Verification items for this drawing (mm, ordinates from the low corner). A direction names the side the tool comes from. Round coordinates to 2 decimals unless told otherwise and drop trailing zeros. Order: outer loops, then holes, each group sorted by start corner. A loop starts at its lowest first (then second) coordinate and runs counter-clockwise, first axis right, second up. Notation, with made-up numbers: (61, 29.25) - (67, 29.25) arc R14 cw to (67, 50.25) - close; hole circle Ø2 at (14.25, 42.25). An arc over 180 degrees is marked (long way). Use a Markdown table: item, result. Add a question column.
(1) Section check B-B on y = 39.5. Record the boundary of the cut face in (x, z).
(2) Section check D-D on x = 31. Record the boundary of the cut face in (y, z).
(3) Gauge pin test, flat ends, axial feed: P1, Ø1.5, axis at y = 55.5, z = 19, coming from the +X side; P2, Ø3, axis at x = 38, y = 24, coming from the -Z side. Record the tip position at first contact, or that the pin passes through.
(4) Mould release check, pull along Y, two halves, no side actions. Record for the marked faces 3, 4 and 5: released by +Y, released by -Y, zero draft, split by the parting line, or undercut.
(5) Section check C-C on z = 2.75. Record the boundary of the cut face in (x, y).
(6) Thickness scan on line 1 along Z through (x, y) = (31, 1); line 2 along Y through (x, z) = (12, 3.5); line 3 along Y through (x, z) = (5, 22.35). Record the ranges inside material, lowest first. Write a range as [from, to].
(7) Section check A-A on x = 7.5. Record the boundary of the cut face in (y, z).
(8) Access from +Z, -Z, +X, -X, +Y, -Y to the whole of each face (thin tool, end or side, straight path). Record for the marked faces 1 and 2.
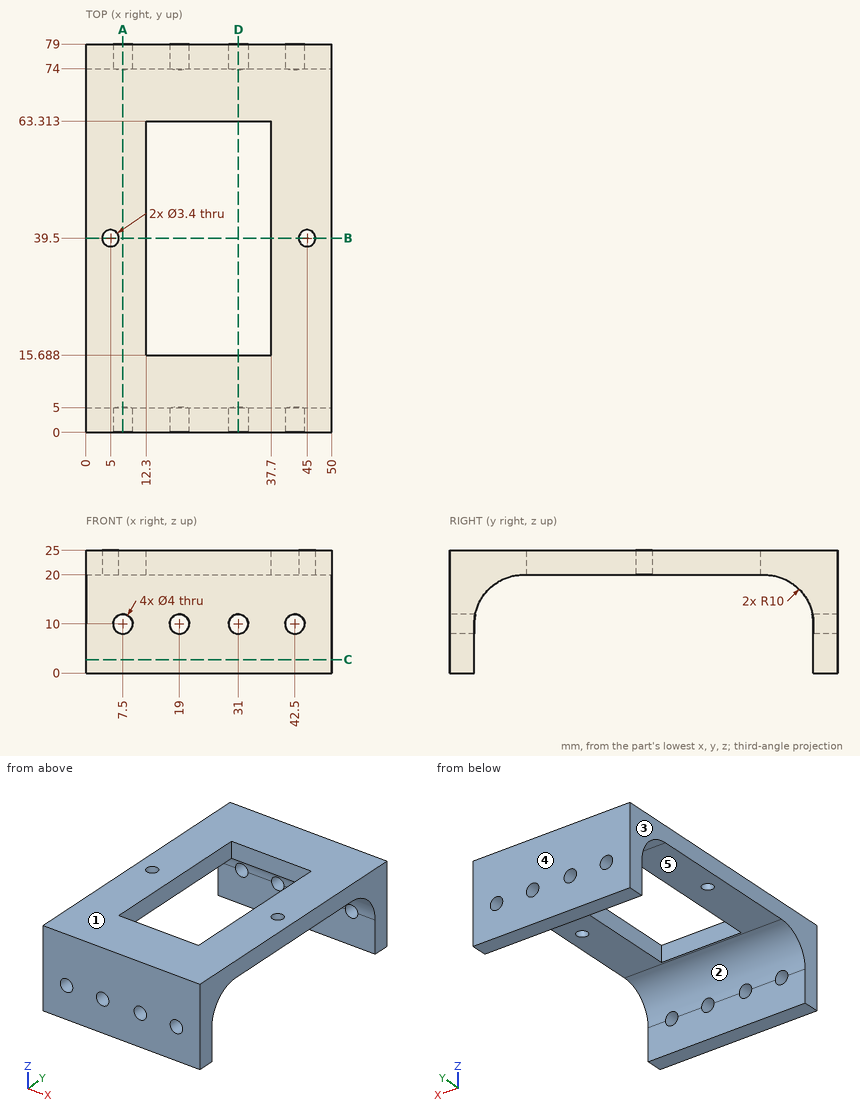
Check sheet entries:
| question | item | result |
|---|---|---|
| 1 | outline | (0, 20) - (3.3, 20) - (3.3, 25) - (0, 25) - close; (6.7, 20) - (12.3, 20) - (12.3, 25) - (6.7, 25) - close; (37.7, 20) - (43.3, 20) - (43.3, 25) - (37.7, 25) - close; (46.7, 20) - (50, 20) - (50, 25) - (46.7, 25) - close |
| 2 | outline | (0, 0) - (5, 0) - (5, 8) - (0, 8) - close; (0, 12) - (5.2, 12) arc R10 cw to (15, 20) - (15.69, 20) - (15.69, 25) - (0, 25) - close; (63.31, 20) - (64, 20) arc R10 cw to (73.8, 12) - (79, 12) - (79, 25) - (63.31, 25) - close; (74, 0) - (79, 0) - (79, 8) - (74, 8) - close |
| 3 | P1 | passes through |
| 3 | P2 | stops at z = 20 |
| 4 | face 3 | zero draft |
| 4 | face 4 | released by +Y |
| 4 | face 5 | undercut |
| 5 | outline | (0, 0) - (50, 0) - (50, 5) - (0, 5) - close; (0, 74) - (50, 74) - (50, 79) - (0, 79) - close |
| 6 | line 1 | z = [0, 8], [12, 25] |
| 6 | line 2 | y = [0, 5], [74, 79] |
| 6 | line 3 | y = [0, 37.8], [41.2, 79] |
| 7 | outline | (0, 0) - (5, 0) - (5, 8) - (0, 8) - close; (0, 12) - (5.2, 12) arc R10 cw to (15, 20) - (64, 20) arc R10 cw to (73.8, 12) - (79, 12) - (79, 25) - (0, 25) - close; (74, 0) - (79, 0) - (79, 8) - (74, 8) - close |
| 8 | face 1 | +Z, +X, -X, +Y, -Y |
| 8 | face 2 | -Z, +X, -X |
